Source: CAD feature listing. Evaluate the final solid. Frame: model axes, mm. Face numbers are marked on the shaded views. A direction names the side the tool comes from. Round coordinates to 2 decimals unless told otherwise and drop trailing zeros. Order: outer loops, then holes, each group sorted by start corner. A loop starts at its lowest first (then second) coordinate and runs counter-clockwise, first axis right, second up. Notation, with made-up numbers: (67.25, 63.5) - (96.25, 63.5) arc R8 cw to (96.25, 72.5) - close; hole circle Ø8 at (22, 63.5). An arc over 180 degrees is marked (long way). Return JSON: item names as keys, results as strings. Group by question number.
1) Contact query for flat-ended pins moving along their axis: P1, Ø1.5, axis at y = -0.5, z = 5, coming from the +X side; P2, Ø2, axis at y = -1, z = 4, coming from the -X side; P3, Ø0.5, axis at x = 0, y = 1.5, coming from the +Z side. Output: stop coordinate, or through.
2) Section A-A, the plane z = 10. Return loops of the section in (x, y), plus the area to 3 significant figures.
3) Ray query, line 1 (Z direction, x = 1.15, y = -0.3); line 2 (Y direction, x = -0.1, z = 5.5); line 3 (Z direction, x = -1.8, y = 0.2). Return the intervals inside material, ascending. Write a range as from..to.
4) Access query for the marked faces 1 and 2. Directions: +Z, -Z, +X, -X, +Y, -Y. A direction counts if a zero-diameter tool reaches every point of the face in a straight line with its end or side. Return the directions, or none.
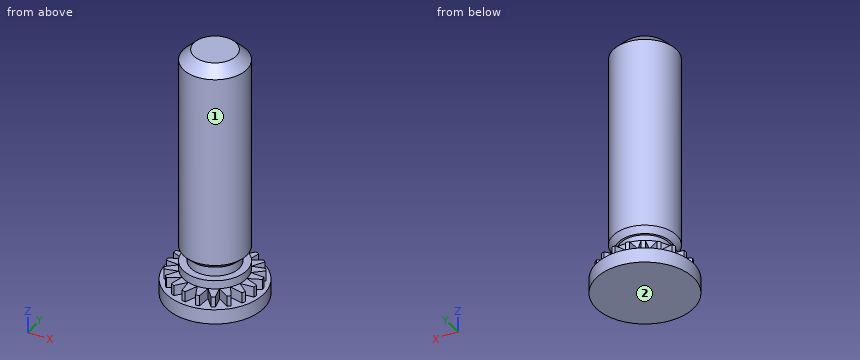
```python
from build123d import *

# Parameters (mm, degrees)
SKETCH_1_R               = 2.3
EXTRUDE_1_DEPTH          = 1.2
SKETCH_2_R               = 1.5
EXTRUDE_2_DEPTH          = 1.5
CUT_EXTRUDE_1_DEPTH      = 0.5
PATTERN_CIRCULAR_1_COUNT = 20
SKETCH_4_W               = 0.35
SKETCH_4_H               = 0.5
SKETCH_6_W               = 9.3
SKETCH_6_H               = 1.5
CHAMFER_2_SIZE           = 0.5
CUT_EXTRUDE_START        = -0.5
SKETCH_7_R               = 2.3
SKETCH_7_R_2             = 2.1
CUT_EXTRUDE_2_DEPTH      = 0.5


with BuildPart() as part:
    # Эскиз1 → Вытянуть1 (new body)
    with BuildSketch(Plane.XY):
        Circle(SKETCH_1_R)
    extrude(amount=EXTRUDE_1_DEPTH)

    # Эскиз2 → Вытянуть2 (add)
    with BuildSketch(Plane.XY.offset(1.2)):
        Circle(SKETCH_2_R)
    extrude(amount=EXTRUDE_2_DEPTH)

    # Эскиз3 → Вырез-Вытянуть1 (cut)
    with BuildSketch(Plane.XY.offset(1.2)):
        Polygon((-0.33137085, 2.3), (0.33137085, 2.3), (0, 1.5), align=None)
    cut_extrude_1 = extrude(amount=-CUT_EXTRUDE_1_DEPTH, mode=Mode.SUBTRACT)

    # Круговой массив1: Вырез-Вытянуть1 ×20 about axis
    pattern_circular_1_axis = Axis((0, 0, 0), (0, 0, 1))
    for i in range(1, PATTERN_CIRCULAR_1_COUNT):
        add(cut_extrude_1.rotate(pattern_circular_1_axis, i * 360 / PATTERN_CIRCULAR_1_COUNT), mode=Mode.SUBTRACT)

    # Эскиз4 → Вырез-Повернуть1 (revolve, cut)
    with BuildSketch(Plane(origin=(0, 0, 0), x_dir=(1, 0, 0), z_dir=(0, 1, 0))):
        with Locations((1.325, -1.85)):
            Rectangle(SKETCH_4_W, SKETCH_4_H)
    revolve(axis=Axis((0, 0, 10.642619983), (0, 0, -1)), mode=Mode.SUBTRACT)

    # Эскиз6 → Повернуть1 (revolve)
    with BuildSketch(Plane(origin=(0, 0, 0), x_dir=(0, 0, -1), z_dir=(1, 0, 0)), mode=Mode.PRIVATE) as revolve_1_sk:
        with Locations((-7.35, -0.75)):
            Rectangle(SKETCH_6_W, SKETCH_6_H)
    revolve(revolve_1_sk.sketch.rotate(Axis((0, 0, 2.7), (0, 0, 1)), 278.047567557), axis=Axis((0, 0, 2.7), (0, 0, 1)))

    # Фаска2
    # the kernel refuses this chamfer: 0.5 mm, written as the material it takes off along each edge
    with BuildSketch(Plane(origin=(0, 0, 12), x_dir=(-0.9901521845161062, -0.1399951838385265, 0), z_dir=(-0.1399951838385265, 0.9901521845161062, 0))) as chamfer_2_piece_1:
        Polygon((1.5, -CHAMFER_2_SIZE), (1.5 - CHAMFER_2_SIZE, 0), (1.5, 0), align=None)
    revolve(axis=Axis((0, 0, 12), (0, 0, 1)), mode=Mode.SUBTRACT)

    # Эскиз7 → Вырез-Вытянуть2 (cut)
    with BuildSketch(Plane.XY.offset(1.2).offset(CUT_EXTRUDE_START)):
        with Locations(Location((0, 0, 0), (0, 0, 180))):
            Circle(SKETCH_7_R)
        Circle(SKETCH_7_R_2, mode=Mode.SUBTRACT)
    extrude(amount=CUT_EXTRUDE_2_DEPTH, mode=Mode.SUBTRACT)

    # Фаска3
    # the kernel refuses this chamfer: 0.25 mm, written as the material it takes off along each edge
    with BuildSketch(Plane(origin=(0, 0, 2.1), x_dir=(1, 0, 0), z_dir=(0, 1, 0))) as chamfer_3_piece_1:
        with BuildLine():
            Line((1.242928932, 0.007071068), (1.507071068, -0.257071068))
            Line((1.507071068, -0.257071068), (1.512071068, -0.257071068))
            ThreePointArc((1.512071068, -0.257071068), (1.505, -0.128535534), (1.505, 0))
            Line((1.505, 0), (1.5, 0.005))
            ThreePointArc((1.5, 0.005), (1.371464466, 0.005), (1.242928932, 0.012071068))
            Line((1.242928932, 0.012071068), (1.242928932, 0.007071068))
        make_face()
    revolve(axis=Axis((0, 0, 2.1), (0, 0, -1)), mode=Mode.SUBTRACT)


solid = part.part
```
Geometry check:
{
 "1": {"P1": "x = 1.5", "P2": "x = -1.5", "P3": "z = 11.75"},
 "2": {"outline": "circle Ø3 at (0, 0)", "area": "7.07 mm2"},
 "3": {"line 1": "0..1.6, 2.1..11.81", "line 2": "-1.5..1.5", "line 3": "0..1.2"},
 "4": {"face 1": "+Z", "face 2": "-Z, +X, -X, +Y, -Y"}
}
